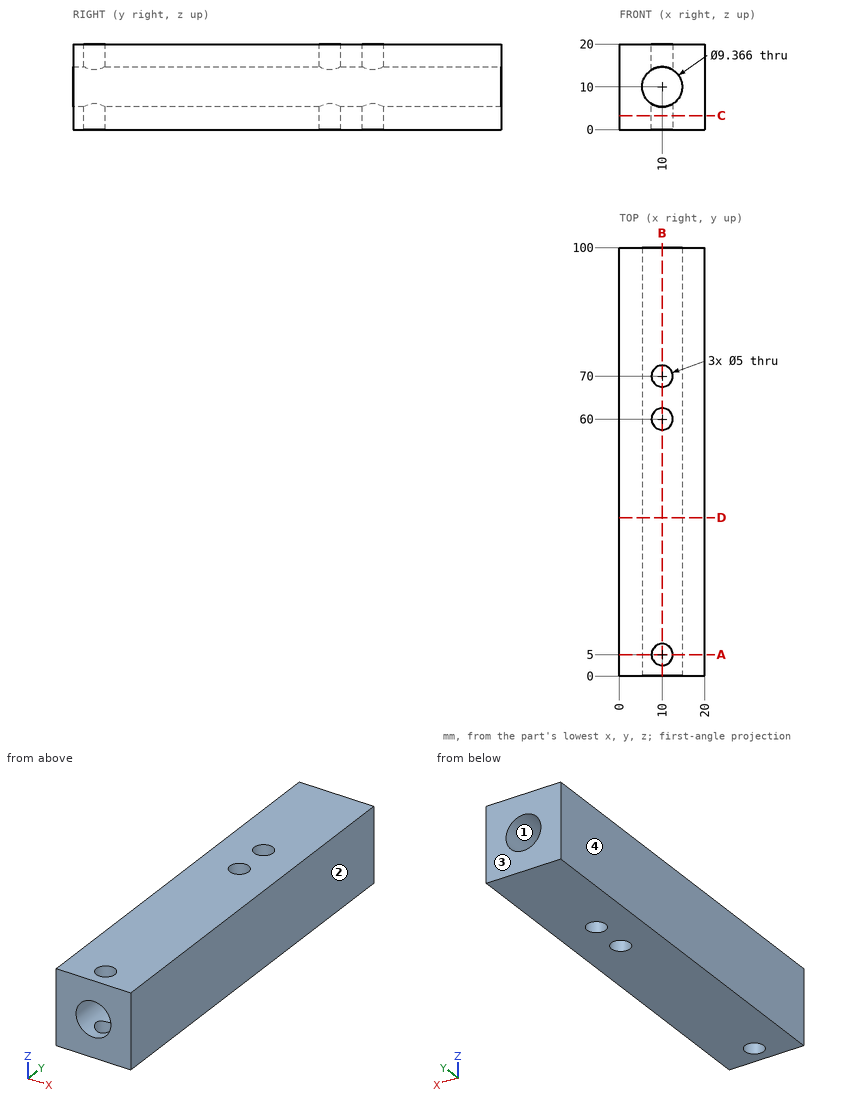
Print and shaded views of the part. All mm, measured from the part's lowest x, y and z. Round coordinates to 2 decimals unless told otherwise and drop trailing zeros. Write each loop counter-clockwise with the first axis right and the second up, starting at its lowest first coordinate (ties: lowest second). Pieces come first, ordered by that corner, then holes.
Item 1: Two-plate mould, pull along X, no slides. Class the marked faces 1, 2, 3 and 4: +X half, -X half, draft (parallel to the pull), parting line (faces both ways), or undercut.
Results:
face 1: undercut
face 2: +X half
face 3: draft
face 4: -X half
Item 2: Cut at D-D, the plane y = 37. Give the cut face in (x, z), plus the area to 3 significant figures.
Results:
outline: (0, 0) - (20, 0) - (20, 20) - (0, 20) - close; hole circle Ø9.37 at (10, 10)
area: 331 mm2
Item 3: Cut at C-C, the plane z = 3.25. Give the cut face in (x, y), plus the area to 3 significant figures.
Results:
outline: (0, 0) - (20, 0) - (20, 100) - (0, 100) - close; hole circle Ø5 at (10, 5); hole circle Ø5 at (10, 60); hole circle Ø5 at (10, 70)
area: 1,940 mm2
Item 4: Probe L1, parallel to Y at x = 10, z = 18.5; L2, parallel to X at y = 10, z = 10.25; L3, parallel to Y at x = 8.5, z = 14.5. List the from-to ranges inside material, lowest first.
Results:
L1: y = 0 to 2.5, 7.5 to 57.5, 62.5 to 67.5, 72.5 to 100
L2: x = 0 to 5.32, 14.68 to 20
L3: y = 0 to 3, 7 to 58, 62 to 68, 72 to 100
Item 5: Cut at A-A, the plane y = 5. Give the cut face in (x, z).
Results:
outline: (0, 0) - (7.5, 0) - (7.5, 6.04) arc R4.68 cw to (7.5, 13.96) - (7.5, 20) - (0, 20) - close; (12.5, 0) - (20, 0) - (20, 20) - (12.5, 20) - (12.5, 13.96) arc R4.68 cw to (12.5, 6.04) - close
Item 6: Cut at B-B, the plane x = 10. Count the separate pieces of the cut face and the enclosed holes in it, plus the area to 3 significant figures.
Results:
separate pieces: 8
enclosed holes: 0
area: 904 mm2
Item 7: Drop a flat-ended pin along its axis: pin 1 Ø6 at (x, z) = (11, 9.5) entering from -Y. Give the stop position or say it passes through.
Results:
pin 1: passes through
